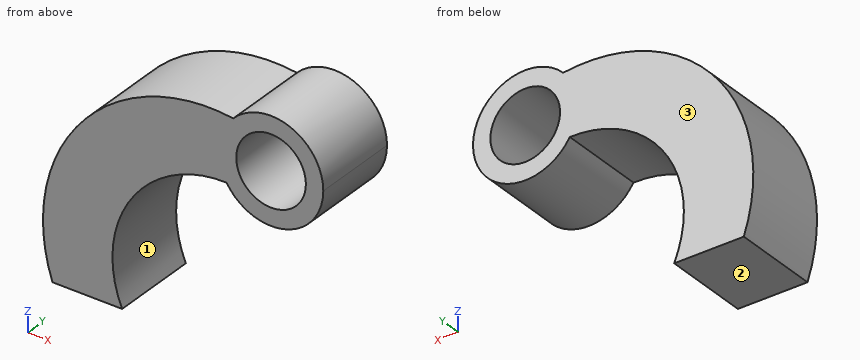
```python
from build123d import *

# Parameters (mm, degrees)
F0_R     = 10
F1_DEPTH = 25


with BuildPart() as f1:
    # F0 (on Front) → F1 (new body)
    with BuildSketch(Plane.XZ):
        with BuildLine():
            ThreePointArc((-12.792136, -7.833343), (-14.916387, 1.581581), (-10.865039, 10.341708))
            ThreePointArc((-10.865039, 10.341708), (-54.658742, -6.783931), (-62.775411, -53.101266))
            Line((-62.775411, -53.101266), (-42.775411, -53.101266))
            ThreePointArc((-42.775411, -53.101266), (-40.200011, -22.243392), (-12.792136, -7.833343))
        make_face()
        with BuildLine():
            ThreePointArc((-12.792136, -7.833343), (4.069273, -14.437487), (15, 0))
            ThreePointArc((15, 0), (5.56886, 13.92795), (-10.865039, 10.341708))
            ThreePointArc((-10.865039, 10.341708), (-14.916387, 1.581581), (-12.792136, -7.833343))
        make_face()
        Circle(F0_R, mode=Mode.SUBTRACT)
    extrude(amount=F1_DEPTH)


solid = f1.part
```
CAD build for the part. Positions are in the model's coordinates, mm. Face numbers are marked on the shaded views. Round coordinates to 2 decimals unless told otherwise and drop trailing zeros. Write each loop counter-clockwise with the first axis right and the second up, starting at its lowest first coordinate (ties: lowest second). Pieces come first, ordered by that corner, then holes. Notation, with made-up numbers: (9, 0) - (52, 0) arc R31 ccw to (52, 33) - close; hole circle Ø6 at (-27.5, 84.5). An arc over 180 degrees is marked (long way). Return JSON: item names as keys, results as strings. Group by question number.
Item 1: Band-saw the part on D-D on x = -16. List the corners of the cut face in (y, z).
Item 2: Mould opens along Z. For the marked faces 1, 2 and 3 say: +Z half, -Z half, draft (parallel to the pull), parting line (faces both ways), or undercut.
Item 3: Probe probe 1 along Z at (x, y) = (0, -17.5); probe 2 along Z at (x, y) = (-55.5, -5); probe 3 along Z at (x, y) = (-11, -4.75). List the from-to ranges inside material, lowest first.
Item 4: Band-saw the part on C-C on y = -9.75. List the corners of the cut face in (x, z), plus the area to 3 significant figures.
Item 5: Flat gauge pins, fed straight in: pin 1 Ø1.5 at (y, z) = (-6, -32) entering from +X; pin 2 Ø2 at (y, z) = (-3.5, -19) entering from -X; pin 3 Ø1.5 at (x, y) = (-5, -9.5) entering from -Z. Where does each tip first touch, or does it go through?
Item 6: Band-saw the part on B-B on z = 2. List the corners of the cut face in (x, y), plus the area to 3 significant figures.
Item 7: Band-saw the part on A-A on x = 0. List the corners of the cut face in (y, z).
Resolved:
{
 "1": {"outline": "(-25, -7.94) - (0, -7.94) - (0, 10.78) - (-25, 10.78) - close"},
 "2": {"face 1": "undercut", "face 2": "-Z half", "face 3": "draft"},
 "3": {"probe 1": "z = -15 to -10, 10 to 15", "probe 2": "z = -53.1 to -7.84", "probe 3": "z = -10.2 to 10.36"},
 "4": {"outline": "(-62.78, -53.1) - (-42.78, -53.1) arc R32.19 cw to (-12.79, -7.83) arc R15 ccw (long way) to (-10.87, 10.34) arc R47.97 ccw to start; hole circle Ø20 at (0, 0)", "area": "1,980 mm²"},
 "5": {"pin 1": "stops at x = -44.34", "pin 2": "stops at x = -62.33", "pin 3": "stops at z = -14.39"},
 "6": {"outline": "(-45.24, -25) - (-9.8, -25) - (-9.8, 0) - (-45.24, 0) - close; (9.8, -25) - (14.87, -25) - (14.87, 0) - (9.8, 0) - close", "area": "1,010 mm²"},
 "7": {"outline": "(-25, -15) - (0, -15) - (0, -10) - (-25, -10) - close; (-25, 10) - (0, 10) - (0, 15) - (-25, 15) - close"}
}
